from build123d import *

# Parameters (mm, degrees)
SKETCH_1_R           = 45
EXTRUDE_1_DEPTH      = 15
SKETCH_6_R           = 10
CUT_EXTRUDE_5_DEPTH  = 26
SKETCH_7_R           = 2.2
CUT_EXTRUDE_6_DEPTH  = 66.383484153
CUT_EXTRUDE_7_DEPTH  = 66.383484153
SKETCH_9_R           = 3.25
CUT_EXTRUDE_8_DEPTH  = 69.92024376
SKETCH_11_R          = 4
CUT_EXTRUDE_9_DEPTH  = 9
CUT_EXTRUDE_START    = -4
CUT_EXTRUDE_10_DEPTH = 4


with BuildPart() as part:
    # 草图1 → 凸台-拉伸1 (new body)
    with BuildSketch(Plane.XY):
        Circle(SKETCH_1_R)
    extrude(amount=EXTRUDE_1_DEPTH)

    # 草图6 → 切除-拉伸5 (cut)
    with BuildSketch(Plane.XY.offset(15)):
        Circle(SKETCH_6_R)
    extrude(amount=-CUT_EXTRUDE_5_DEPTH, mode=Mode.SUBTRACT)

    # 草图7 → 切除-拉伸6 (cut, through all)
    with BuildSketch(Plane.XY.offset(15)):
        with Locations((17.25, 0)):
            Circle(SKETCH_7_R)
        with Locations((8.625, -14.938938215)):
            Circle(SKETCH_7_R)
        with Locations((-8.625, -14.938938215)):
            Circle(SKETCH_7_R)
        with Locations((-17.25, 0)):
            Circle(SKETCH_7_R)
        with Locations((-8.625, 14.938938215)):
            Circle(SKETCH_7_R)
        with Locations((8.625, 14.938938215)):
            Circle(SKETCH_7_R)
    extrude(amount=-CUT_EXTRUDE_6_DEPTH, mode=Mode.SUBTRACT)

    # 草图8 → 切除-拉伸7 (cut, through all)
    with BuildSketch(Plane.XY.offset(15)):
        with BuildLine():
            ThreePointArc((-25, 37.416573868), (-45, 0), (-25, -37.416573868))
            Line((-25, -37.416573868), (-25, 37.416573868))
        make_face()
        with BuildLine():
            Line((25, 37.416573868), (25, -37.416573868))
            ThreePointArc((25, -37.416573868), (39.686269666, -21.213203436), (45, 0))
            ThreePointArc((45, 0), (39.686269666, 21.213203436), (25, 37.416573868))
        make_face()
    extrude(amount=-CUT_EXTRUDE_7_DEPTH, mode=Mode.SUBTRACT)

    # 草图9 → 切除-拉伸8 (cut, through all)
    with BuildSketch(Plane(origin=(25, 0, 0), x_dir=(0, 0, -1), z_dir=(1, 0, 0))):
        with Locations((-6, 23.45)):
            Circle(SKETCH_9_R)
        with Locations((-6, -23.63)):
            Circle(SKETCH_9_R)
    extrude(amount=-CUT_EXTRUDE_8_DEPTH, mode=Mode.SUBTRACT)

    # 草图11 → 切除-拉伸9 (cut)
    with BuildSketch(Plane(origin=(0, 0, 0), x_dir=(-1, 0, 0), z_dir=(0, 0, -1))):
        with Locations((-8.625, 14.938938215)):
            Circle(SKETCH_11_R)
        with Locations((-17.25, 0)):
            Circle(SKETCH_11_R)
        with Locations((-8.625, -14.938938215)):
            Circle(SKETCH_11_R)
        with Locations((8.625, 14.938938215)):
            Circle(SKETCH_11_R)
        with Locations((8.625, -14.938938215)):
            Circle(SKETCH_11_R)
        with Locations((17.25, 0)):
            Circle(SKETCH_11_R)
    extrude(amount=-CUT_EXTRUDE_9_DEPTH, mode=Mode.SUBTRACT)

    # 草图13 → 切除-拉伸10 (cut)
    with BuildSketch(Plane.XY.offset(15).offset(CUT_EXTRUDE_START)):
        with BuildLine():
            ThreePointArc((25, 37.416573868), (0, 45), (-25, 37.416573868))
            Line((-25, 37.416573868), (-25, 2.6e-08))
            ThreePointArc((-25, 2.6e-08), (1.3e-08, 25), (25, 0))
            Line((25, 0), (25, 37.416573868))
        make_face()
        with BuildLine():
            ThreePointArc((25, 0), (-1.3e-08, -25), (-25, 2.6e-08))
            Line((-25, 2.6e-08), (-25, -37.416573868))
            ThreePointArc((-25, -37.416573868), (0, -45), (25, -37.416573868))
            Line((25, -37.416573868), (25, 0))
        make_face()
    extrude(amount=CUT_EXTRUDE_10_DEPTH, mode=Mode.SUBTRACT)


solid = part.part
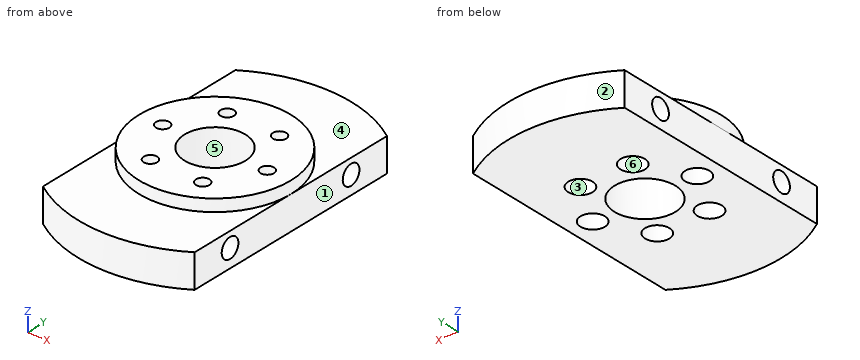
Read the model definition and answer for the solid it produces. Units are mm, in the model's axes. Face numbers are marked on the shaded views. A direction names the side the tool comes from. Round coordinates to 2 decimals unless told otherwise and drop trailing zeros. Write each loop counter-clockwise with the first axis right and the second up, starting at its lowest first coordinate (ties: lowest second). Pieces come first, ordered by that corner, then holes.
Q1. Straight lines are drawn through the part: line 1 (Y direction, x = -0.5, z = 6); line 2 (Y direction, x = 7.5, z = 12); line 3 (X direction, y = -13, z = 3.25). For each, find the intervals that lie inside material, in ascending order.
Values:
line 1: y = -45 to -26.88, -20.38 to -9.99, 9.99 to 20.2, 26.7 to 45
line 2: y = -23.85 to -16.83, -13.05 to -6.61, 6.61 to 13.05, 16.83 to 23.85
line 3: x = -25 to -12.12, -5.13 to 5.13, 12.12 to 25
Q2. A tool of negligible diameter and unlimited length cuts with its end or side. For the marked faces 5 and 6, from which of +Z, -Z, +X, -X, +Y, -Y can it reach the whole face along a straight path? Write none if from no direction.
Values:
face 5: +Z, -Z
face 6: -Z
Q3. The mould has two halves that part along X. Classify the marked faces 1, 2, 3 and 4: released by +X, released by -X, zero draft, split by the parting line, or undercut.
Values:
face 1: released by +X
face 2: split by the parting line
face 3: undercut
face 4: zero draft
Q4. Find section C-C on y = -5. Determine the outline of the cut face in (x, z).
Values:
outline: (-25, 0) - (-8.66, 0) - (-8.66, 15) - (-24.49, 15) - (-24.49, 11) - (-25, 11) - close; (8.66, 0) - (25, 0) - (25, 11) - (24.49, 11) - (24.49, 15) - (8.66, 15) - close
Q5. Find section D-D on z = 13.5. Determine the outline of the cut face in (x, y) (3 decimals), and give its area (3 significant figures).
Values:
outline: circle Ø50 at (0, 0); hole circle Ø4.4 at (-17.25, 0); hole circle Ø4.4 at (-8.625, -14.939); hole circle Ø4.4 at (-8.625, 14.939); hole circle Ø20 at (0, 0); hole circle Ø4.4 at (8.625, -14.939); hole circle Ø4.4 at (8.625, 14.939); hole circle Ø4.4 at (17.25, 0)
area: 1,560 mm2
Q6. Find section A-A on x = 0. Determine the outline of the cut face in (y, z), and give its area (3 significant figures).
Values:
outline: (-45, 0) - (-10, 0) - (-10, 15) - (-25, 15) - (-25, 11) - (-45, 11) - close; (10, 0) - (45, 0) - (45, 11) - (25, 11) - (25, 15) - (10, 15) - close; hole circle Ø6.5 at (-23.63, 6); hole circle Ø6.5 at (23.45, 6)
area: 824 mm2
Q7. Flat-ended cylindrical pins translate along their axes: P1, Ø1, axis at x = 5, z = 5.5, coming from the +Y side; P2, Ø1.5, axis at x = 4, y = -19.5, coming from the -Z side; P3, Ø8, axis at x = 8, z = 1.5, coming from the -Y side; P4, Ø4, axis at x = 7.5, y = -16.5, coming from the -Z side. Find the tip coordinate at first contact, or state that the pin passes through.
Values:
P1: stops at y = 44.77
P2: stops at z = 0
P3: stops at y = -44.82
P4: stops at z = 9
Q8. Find section B-B on z = 4. State how many separate pieces and enclosed holes the cut face has, and give its area (3 significant figures).
Values:
separate pieces: 3
enclosed holes: 7
area: 3,130 mm2
